Can you work these out from the drawing? Everything is in mm from the part's minimum corner. Give positions to 0.01 mm unless a question says otherwise; leave off trailing zeros. Write each loop counter-clockwise with the first axis right and the second up, starting at its lowest first coordinate (ties: lowest second). Pieces come first, ordered by that corner, then holes. Notation, with made-up numbers: (52.5, 85) -> (91.5, 85) arc R16 cw to (91.5, 112) -> close; hole circle Ø3 at (7, -16.75). An arc over 180 degrees is marked (long way). Return JSON: item names as keys, results as strings.
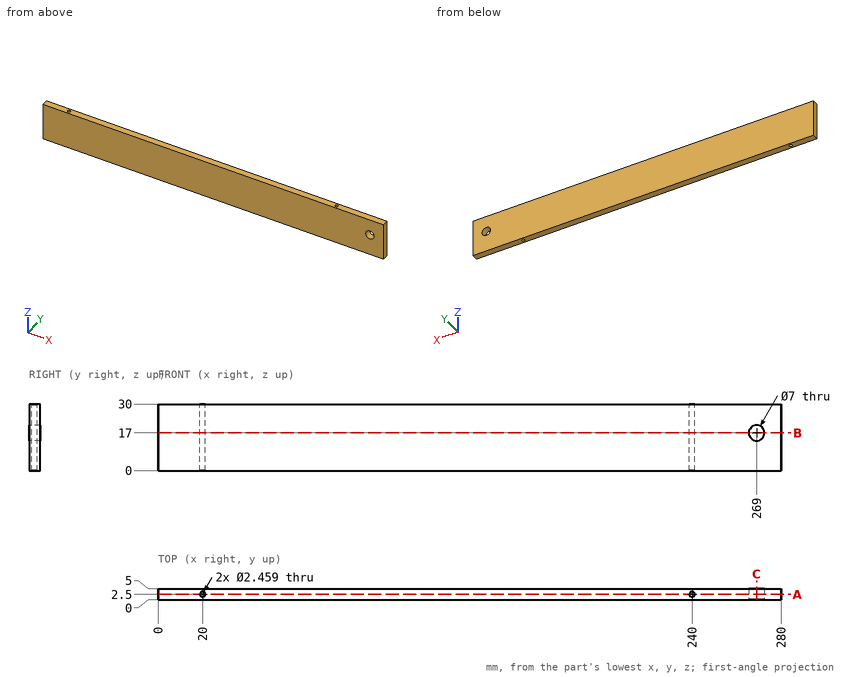
1. Suppose I cut it at B-B, the plane z = 17. List the corners of the cut face in (x, y) for me.
Taken from the geometry:
{"outline": "(0, 0) -> (265.5, 0) -> (265.5, 5) -> (0, 5) -> close; (272.5, 0) -> (280, 0) -> (280, 5) -> (272.5, 5) -> close; hole circle Ø2.46 at (20, 2.5); hole circle Ø2.46 at (240, 2.5)"}
2. Suppose I cut it at A-A, the plane y = 2.5. List the corners of the cut face in (x, z) for me.
Taken from the geometry:
{"outline": "(0, 0) -> (18.77, 0) -> (18.77, 30) -> (0, 30) -> close; (21.23, 0) -> (238.77, 0) -> (238.77, 30) -> (21.23, 30) -> close; (241.23, 0) -> (280, 0) -> (280, 30) -> (241.23, 30) -> close; hole circle Ø7 at (269, 17)"}
3. For pin 1 Ø5.5 at (x, z) = (269, 17) entering from +Y, with a flat end and sliding along its axis, tell me the tip position at first contact or that it passes through.
Taken from the geometry:
{"pin 1": "passes through"}
4. Suppose I cut it at C-C, the plane x = 269. List the corners of the cut face in (y, z) for me, and give its area (3 significant figures).
Taken from the geometry:
{"outline": "(0, 0) -> (5, 0) -> (5, 13.5) -> (0, 13.5) -> close; (0, 20.5) -> (5, 20.5) -> (5, 30) -> (0, 30) -> close", "area": "115 mm²"}
5. If I drill on line 1 (X direction, y = 2.2, z = 26); line 2 (Y direction, x = 240, z = 8); line 3 (X direction, y = 1.9, z = 12.75), over which ranges is the centre line in solid material (lowest first)? Write a range as [from, to].
Taken from the geometry:
{"line 1": "x = [0, 18.81], [21.19, 238.81], [241.19, 280]", "line 2": "y = [0, 1.27], [3.73, 5]", "line 3": "x = [0, 18.93], [21.07, 238.93], [241.07, 280]"}
